```python
from build123d import *

# Parameters (mm, degrees)
SKETCH2_R                  = 3.15
CUT_EXTRUDE1_DEPTH         = 18.109938632
M2X0_4_TAPPED_HOLE2_REACH  = 21.513
M2X0_4_TAPPED_HOLE2_BORE_R = 0.8


with BuildPart() as part:
    # Sketch1 → Revolve1 (revolve)
    with BuildSketch(Plane.XY, mode=Mode.PRIVATE) as revolve1_sk:
        with BuildLine():
            Line((-10.5, -3), (-5, -3))
            Line((-5, -3), (-5, -5.5))
            Line((-5, -5.5), (0, -5.5))
            Line((0, -5.5), (0, 3))
            Line((0, 3), (-10.5, 3))
            Line((-10.5, 3), (-10.5, 2.38125))
            Line((-10.5, 2.38125), (-9.5, 2.38125))
            ThreePointArc((-9.5, 2.38125), (-7.11875, 0), (-9.5, -2.38125))
            Line((-9.5, -2.38125), (-10.5, -2.38125))
            Line((-10.5, -2.38125), (-10.5, -3))
        make_face()
    revolve(revolve1_sk.sketch.rotate(Axis((0, 5.888182105, 0), (0, -1, 0)), 270), axis=Axis((0, 5.888182105, 0), (0, -1, 0)))

    # Sketch2 → Cut-Extrude1 (cut, through all)
    with BuildSketch(Plane(origin=(0, 3, 0), x_dir=(1, 0, 0), z_dir=(0, 1, 0))):
        with Locations(Location((0, 0, 0), (0, 0, 270))):
            Circle(SKETCH2_R)
    extrude(amount=-CUT_EXTRUDE1_DEPTH, mode=Mode.SUBTRACT)

    # M2x0.4 Tapped Hole2 bore → M2x0.4 Tapped Hole2 (cut, up to next)
    with BuildSketch(Plane(origin=(5, 0, 0), x_dir=(0, 0, -1), z_dir=(1, 0, 0)), mode=Mode.PRIVATE) as m2x0_4_tapped_hole2_sk1:
        with Locations((0, -4.25)):
            Circle(M2X0_4_TAPPED_HOLE2_BORE_R)
    m2x0_4_tapped_hole2_tool1 = extrude(m2x0_4_tapped_hole2_sk1.sketch, amount=-M2X0_4_TAPPED_HOLE2_REACH, mode=Mode.PRIVATE) & part.part
    add(m2x0_4_tapped_hole2_tool1.solids().sort_by_distance((5, -4.25, 0))[0], mode=Mode.SUBTRACT)


solid = part.part
```
Work out the finished part from the listing and answer in its coordinate system (mm). A direction names the side the tool comes from. Give positions to 0.01 mm unless a question says otherwise; leave off trailing zeros. Write each loop counter-clockwise with the first axis right and the second up, starting at its lowest first coordinate (ties: lowest second). Pieces come first, ordered by that corner, then holes.
(1) Which of the six approach directions +Z, -Z, +X, -X, +Y, -Y give full straight-line access (tool end or side, diameter ignored) to faces 1 (the flat face through (9, 2.381, -5)), 2 (the cylindrical face through (4.04, -5.03, 0.17)), 3 (the cylindrical face through (4.88, -4.27, -1.08))?
Final values:
face 1: none
face 2: +X
face 3: -Y
(2) The part is cut by section D-D on y = -4.25. Write down the section's boundary in (x, z), plus the area to 3 significant figures.
Final values:
outline: (3.05, -0.8) arc R3.15 cw (long way) to (3.05, 0.8) - (4.94, 0.8) arc R5 ccw (long way) to (4.94, -0.8) - close
area: 44.4 mm2
(3) Straight lines are drawn through the part: line 1 (Y direction, x = 3.55, z = 0); line 2 (Y direction, x = 9.25, z = -3.25); line 3 (Z direction, x = 2.75, y = -1.75). For each, find the intervals that lie inside material, in ascending order.
Final values:
line 1: y = -5.5 to -5.05, -3.45 to 3
line 2: y = -3 to -2.38, 2.38 to 3
line 3: z = -7.39 to -1.54, 1.54 to 7.39
(4) The mould has two halves that part along Z. Classify faces 4 (the cylindrical face through (-3.075, -1.19, -0.683)), 5 (the cylindrical face through (-3.2, -2.7, 10)), 6 (the flat face through (3.3, -5.5, -0.1)): pulls with the +Z half, pulls with the -Z half, needs draft (parallel to the pull), parting line crosses it, or undercut.
Final values:
face 4: undercut
face 5: parting line crosses it
face 6: needs draft
(5) The part is cut by section C-C on y = 0.25. Write down the section's boundary in (x, z), plus the area to 3 significant figures.
Final values:
outline: circle Ø14.26 at (0, 0); hole circle Ø6.3 at (0, 0)
area: 129 mm2
(6) Flat-ended cylindrical pins translate along their axes: pin 1 Ø5 at (x, z) = (0, 0) entering from +Y; pin 2 Ø4 at (x, y) = (-3.5, 0) entering from -Z; pin 3 Ø1.8 at (y, z) = (-4.25, 0) entering from -X; pin 4 Ø1.5 at (y, z) = (0, 0.5) entering from +X. Find the tip coordinate at first contact, or state that the pin passes through.
Final values:
pin 1: passes through
pin 2: stops at z = -7.54
pin 3: stops at x = -5
pin 4: stops at x = 7.23
(7) The part is cut by section A-A on x = 0. Write down the section's boundary in (y, z), plus the area to 3 significant figures.
Final values:
outline: (-5.5, -5) - (-3, -5) - (-3, -10.5) - (-2.38, -10.5) - (-2.38, -9.5) arc R2.38 cw to (2.38, -9.5) - (2.38, -10.5) - (3, -10.5) - (3, -3.15) - (-5.5, -3.15) - close; (-5.5, 3.15) - (3, 3.15) - (3, 10.5) - (2.38, 10.5) - (2.38, 9.5) arc R2.38 cw to (-2.38, 9.5) - (-2.38, 10.5) - (-3, 10.5) - (-3, 5) - (-5.5, 5) - close
area: 70.1 mm2
(8) The part is cut by section B-B on z = 0. Write down the section's boundary in (x, y), plus the area to 3 significant figures.
Final values:
outline: (-10.5, -3) - (-5, -3) - (-5, -5.5) - (-3.15, -5.5) - (-3.15, 3) - (-10.5, 3) - (-10.5, 2.38) - (-9.5, 2.38) arc R2.38 cw to (-9.5, -2.38) - (-10.5, -2.38) - close; (3.15, -5.5) - (5, -5.5) - (5, -5.05) - (3.15, -5.05) - close; (3.15, -3.45) - (5, -3.45) - (5, -3) - (10.5, -3) - (10.5, -2.38) - (9.5, -2.38) arc R2.38 cw to (9.5, 2.38) - (10.5, 2.38) - (10.5, 3) - (3.15, 3) - close
area: 67.2 mm2
